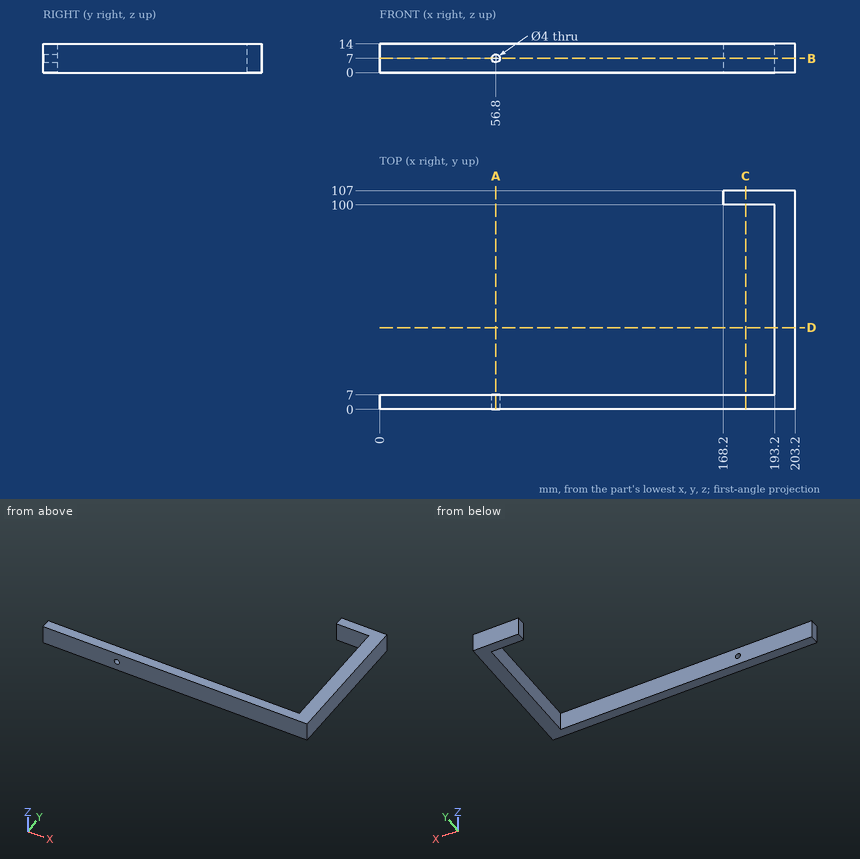
Input: dimensioned drawing with shaded views. Units: mm. Origin: part minimum x, y, z. Give positions to 0.01 mm unless a question says otherwise; leave off trailing zeros. Write each loop counter-clockwise with the first axis right and the second up, starting at its lowest first coordinate (ties: lowest second). Pieces come first, ordered by that corner, then holes.
1. Section query C-C (x = 179). Return the cut outline in (y, z).
2. Section query A-A (x = 56.8). Return the cut outline in (y, z).
3. Section query D-D (y = 40). Return the cut outline in (x, z).
4. Material intervals for line 1 along Z through (x, y) = (56.8, 2); line 2 along X through (y, z) = (1.5, 7); line 3 along Y through (x, z) = (191.5, 4.75), sorted ascending.
5. First-contact query: pin 1 (4 mm diameter, centred on y = 72.5, z = 9.5, fed in from -X); pin 2 (7 mm diameter, centred on x = 73, z = 4, fed in from +Y); pin 3 (3.5 mm diameter, centred on y = 104.5, z = 6.5, fed in from -X). Flat tips, straight axial feed; report the tip coordinate or a pass-through.
6. Section query B-B (z = 7). Return the cut outline in (x, y), then the cut area to 3 significant figures.
Output values:
1. outline: (0, 0) - (7, 0) - (7, 14) - (0, 14) - close; (100, 0) - (107, 0) - (107, 14) - (100, 14) - close
2. outline: (0, 0) - (7, 0) - (7, 5) - (0, 5) - close; (0, 9) - (7, 9) - (7, 14) - (0, 14) - close
3. outline: (193.2, 0) - (203.2, 0) - (203.2, 14) - (193.2, 14) - close
4. line 1: z = 0 to 5, 9 to 14
4. line 2: x = 0 to 54.8, 58.8 to 203.2
4. line 3: y = 0 to 7, 100 to 107
5. pin 1: stops at x = 193.2
5. pin 2: stops at y = 7
5. pin 3: stops at x = 168.2
6. outline: (0, 0) - (54.8, 0) - (54.8, 7) - (0, 7) - close; (58.8, 0) - (203.2, 0) - (203.2, 107) - (168.2, 107) - (168.2, 100) - (193.2, 100) - (193.2, 7) - (58.8, 7) - close
6. area: 2,570 mm2
